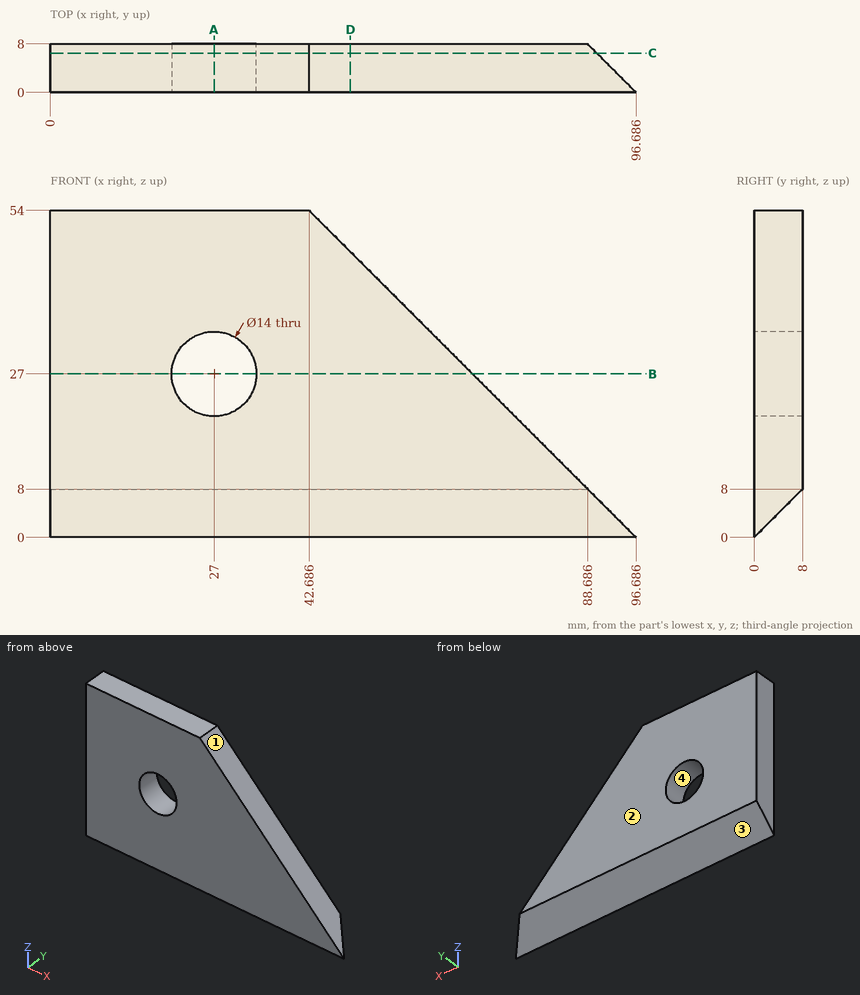
Job drawing, mm, ordinate dimensions from the low corner. One solid piece. Coordinates: 2 decimals unless noted, no trailing zeros. Write each loop counter-clockwise with the first axis right and the second up, starting at its lowest first coordinate (ties: lowest second). Pieces come first, ordered by that corner, then holes. Notation, with made-up numbers: M 79.25,-27 L 119.25,-27 A9 cw 119.25,-19 Z; hole C -35.5,6 d10. An arc over 180 degrees is marked long. Answer as a JSON object with one key per item and string values. Group by question number.
1) Saw through at C-C (y = 6.5). Write the cut outline in (x, z).
2) Wall check: line 1 (Z direction, x = 21, y = 6.5) (1 decimal); line 2 (Z direction, x = 27, y = 3.75); line 3 (X direction, y = 0.5, z = 31) (1 decimal). Give the ranges that are in metal, low to high. Write a range as from..to.
3) Mould opens along Z. For the marked faces 1, 2, 3 and 4 say: +Z half, -Z half, draft (parallel to the pull), parting line (faces both ways), or undercut.
4) Pin check, flat tips, straight feed: pin 1 Ø3 at (x, y) = (81, 6) entering from +Z; pin 2 Ø1.5 at (y, z) = (4, 34.5) entering from +X; pin 3 Ø4 at (y, z) = (2.5, 8) entering from +X. Stop position of each tip, or through.
5) Saw through at A-A (x = 27). Write the cut outline in (y, z).
6) Saw through at B-B (z = 27). Write the cut outline in (x, y).
7) Saw through at D-D (x = 49.5). Write the cut outline in (y, z).
Values follow:
{
 "1": {"outline": "M 0,6.5 L 90.19,6.5 L 42.69,54 L 0,54 Z; hole C 27,27 d14"},
 "2": {"line 1": "z = 6.5..23.4, 30.6..54", "line 2": "z = 3.75..20, 34..54", "line 3": "x = 0..21.3, 32.7..65.7"},
 "3": {"face 1": "+Z half", "face 2": "draft", "face 3": "-Z half", "face 4": "undercut"},
 "4": {"pin 1": "stops at z = 17.19", "pin 2": "stops at x = 62.94", "pin 3": "stops at x = 90.69"},
 "5": {"outline": "M 0,0 L 8,8 L 8,20 L 0,20 Z; M 0,34 L 8,34 L 8,54 L 0,54 Z"},
 "6": {"outline": "M 0,0 L 20,0 L 20,8 L 0,8 Z; M 34,0 L 69.69,0 L 69.69,8 L 34,8 Z"},
 "7": {"outline": "M 0,0 L 8,8 L 8,47.19 L 0,47.19 Z"}
}
